from build123d import *

# Parameters (mm, degrees)
SKETCH_1_R          = 5.5
EXTRUDE_1_DEPTH     = 12
SKETCH_2_R          = 2
CUT_EXTRUDE_1_DEPTH = 12
EXTRUDE_2_DEPTH     = 6
SKETCH_4_R          = 2
CUT_EXTRUDE_2_DEPTH = 21.217986778
SKETCH_5_R          = 2
CUT_EXTRUDE_3_DEPTH = 6


with BuildPart() as part:
    # 草图1 → 凸台-拉伸1 (new body)
    with BuildSketch(Plane(origin=(0, 0, 0), x_dir=(1, 0, 0), z_dir=(0, 1, 0))):
        with Locations(Location((0, 0, 0), (0, 0, 270))):
            Circle(SKETCH_1_R)
    extrude(amount=EXTRUDE_1_DEPTH)

    # 草图2 → 切除-拉伸1 (cut)
    with BuildSketch(Plane(origin=(0, 12, 0), x_dir=(1, 0, 0), z_dir=(0, 1, 0))):
        with Locations(Location((0, 0, 0), (0, 0, 270))):
            Circle(SKETCH_2_R)
    extrude(amount=-CUT_EXTRUDE_1_DEPTH, mode=Mode.SUBTRACT)

    # 草图3 → 凸台-拉伸2 (add)
    with BuildSketch(Plane(origin=(0, 0, 0), x_dir=(-1, 0, 0), z_dir=(0, -1, 0))):
        Polygon((3.577982267, -5.932793852), (6.926941325, 0.132226612), (3.348959058, 6.065020464), (-3.577982267, 5.932793852), (-6.926941325, -0.132226612), (-3.348959058, -6.065020464), align=None)
    extrude(amount=EXTRUDE_2_DEPTH)

    # 草图4 → 切除-拉伸2 (cut, through all)
    with BuildSketch(Plane.XZ.offset(6)):
        with Locations(Location((0, 0, 0), (0, 0, 90))):
            Circle(SKETCH_4_R)
    extrude(amount=-CUT_EXTRUDE_2_DEPTH, mode=Mode.SUBTRACT)

    # 草图5 → 切除-拉伸3 (cut)
    with BuildSketch(Plane(origin=(0.114511605, 0, -5.998907158), x_dir=(-0.9998178596958822, 0, -0.019085267437092362), z_dir=(0.01908526743709236, 0, -0.9998178596958821))):
        with Locations((0, 6)):
            Circle(SKETCH_5_R)
    extrude(amount=-CUT_EXTRUDE_3_DEPTH, mode=Mode.SUBTRACT)


solid = part.part
Check sheet for the modelled part. Datum: model origin and axes. Units: mm. A direction names the side the tool comes from. Give positions to 0.01 mm unless a question says otherwise; leave off trailing zeros. Loops run counter-clockwise (first coordinate to the right, second up) from the corner with the lowest first, then second, coordinate; pieces in that order, holes last. Notation, with made-up numbers: M 67.25,-23 L 87.25,-23 A19 ccw 87.25,10 Z; hole C 19,39.25 d2. An arc over 180 degrees is marked long. Answer as a JSON object with one key per item and string values. Group by question number.
Q1. Release check for a two-part mould opening along X. For faces 1 (the cylindrical face through (-2.11, 5.92, 5.08)), 2 (the cylindrical face through (0.766, 2.874, 1.847)), 3 (the flat face through (5.23, -2.96, -2.94)) record: released by +X, released by -X, zero draft, split by the parting line, or undercut.
Q2. Cross-section at D-D on x = -1. Give the number of separate pieces and of enclosed holes in the cut face, then the cut area to 3 significant figures.
Q3. Material ranges on line 1 along X through (y, z) = (2.75, 0); line 2 along Y through (x, z) = (4.5, -4), recorded low to high. Write a range as [from, to].
Q4. Access from +Z, -Z, +X, -X, +Y, -Y to the whole of each face (thin tool, end or side, straight path). Record for faces 4 (the cylindrical face through (2.063, 6.088, -3.362)), 5 (the flat face through (-5, 0, -3)), 6 (the flat face through (5.16, -2.96, 3.06)).
Q5. Cross-section at C-C on x = 4. Record the cut outline in (y, z), then the cut area to 3 significant figures.
Q6. Go/stop test with flat-tipped pins: P1, Ø1, axis at y = 9, z = 3.5, coming from the +X side; P2, Ø6, axis at x = -0.5, z = -1.5, coming from the +Y side; P3, Ø1.5, axis at x = -2.5, y = 4.5, coming from the +Z side; P4, Ø1.5, axis at y = -4, z = 3.5, coming from the +X side. Record where each tip stops, or that it passes through.
Q7. Cross-section at B-B on z = 5. Record the cut outline in (x, y), then the cut area to 3 significant figures.
Q8. Cross-section at A-A on y = -1.5. Record the cut outline in (x, z), then the cut area to 3 significant figures.
Evaluation:
{
 "1": {"face 1": "split by the parting line", "face 2": "undercut", "face 3": "released by +X"},
 "2": {"separate pieces": "3", "enclosed holes": "0", "area": "127 mm2"},
 "3": {"line 1": "x = [-5.5, -2], [2, 5.5]", "line 2": "y = [-6, 0]"},
 "4": {"face 4": "none", "face 5": "+Y", "face 6": "+Z, +X, +Y, -Y"},
 "5": {"outline": "M -6,-5.17 L 0,-5.17 L 0,-3.77 L 12,-3.77 L 12,3.77 L 0,3.77 L 0,4.99 L -6,4.99 Z", "area": "152 mm2"},
 "6": {"P1": "stops at x = 4.61", "P2": "stops at y = 12", "P3": "stops at z = 5.21", "P4": "stops at x = 5.35"},
 "7": {"outline": "M -4.09,-6 L 3.99,-6 L 3.99,0 L 2.29,0 L 2.29,12 L -2.29,12 L -2.29,0 L -4.09,0 Z", "area": "103 mm2"},
 "8": {"outline": "M -6.93,-0.13 L -3.35,-6.07 L 3.58,-5.93 L 6.93,0.13 L 3.35,6.07 L -3.58,5.93 Z; hole C 0,0 d4", "area": "112 mm2"}
}
